Design review of the part built by this model. Coordinates are the model's own, in mm. Face numbers are marked on the shaded views. A direction names the side the tool comes from. Round coordinates to 2 decimals unless told otherwise and drop trailing zeros. Loops run counter-clockwise (first coordinate to the right, second up) from the corner with the lowest first, then second, coordinate; pieces in that order, holes last. Notation, with made-up numbers: (43, -31.75) -> (93, -31.75) arc R25 ccw to (93, -14.75) -> close; hole circle Ø3 at (-32, -31.75). An arc over 180 degrees is marked (long way). Use a Markdown table: item, result. Add a question column.
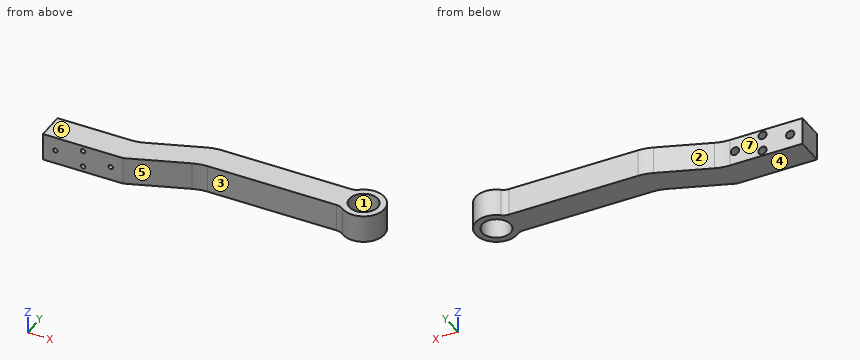
from build123d import *

# Parameters (mm, degrees)
MODEL_R             = 10.3
EXTRUDE_1_DEPTH     = 20
SKETCH_2_R          = 1.6
CUT_EXTRUDE_1_DEPTH = 20
SKETCH_3_R          = 3
CUT_EXTRUDE_2_DEPTH = 8.5


with BuildPart() as part:
    # Model → 凸台-拉伸1 (new body)
    with BuildSketch(Plane.XY):
        with BuildLine():
            Line((125.228900422, 213.510087452), (183.228900422, 213.510087452))
            Line((183.228900422, 213.510087452), (225.242736582, 228.801873242))
            ThreePointArc((225.242736582, 228.801873242), (230.293895552, 230.155327209), (235.503340882, 230.611094618))
            Line((235.503340882, 230.611094618), (328.909813266, 230.611094618))
            ThreePointArc((328.909813266, 230.611094618), (331.547600788, 230.163715156), (333.89036532, 228.871613865))
            ThreePointArc((333.89036532, 228.871613865), (358.22890041, 240.609493061), (333.891295649, 252.349301102))
            ThreePointArc((333.891295649, 252.349301102), (331.548694356, 251.057478239), (328.911168476, 250.610215048))
            Line((328.911168476, 250.610215048), (235.503478715, 250.611047476))
            ThreePointArc((235.503478715, 250.611047476), (230.293897677, 250.15530328), (225.242607062, 248.8018261))
            Line((225.242607062, 248.8018261), (188.1996953, 235.319308829))
            ThreePointArc((188.1996953, 235.319308829), (183.14853633, 233.965854862), (177.939091, 233.510087452))
            Line((177.939091, 233.510087452), (125.228900422, 233.510087452))
            Line((125.228900422, 233.510087452), (125.228900422, 213.510087452))
        make_face()
        with Locations((343.228900422, 240.610087452)):
            Circle(MODEL_R, mode=Mode.SUBTRACT)
    extrude(amount=EXTRUDE_1_DEPTH)

    # 草图2 → 切除-拉伸1 (cut)
    with BuildSketch(Plane.XZ.offset(-213.510087452)):
        with Locations((134.228900422, 10)):
            Circle(SKETCH_2_R)
        with Locations((174.228900422, 10)):
            Circle(SKETCH_2_R)
        with Locations((154.228900422, 16)):
            Circle(SKETCH_2_R)
        with Locations((154.228900422, 4)):
            Circle(SKETCH_2_R)
    extrude(amount=-CUT_EXTRUDE_1_DEPTH, mode=Mode.SUBTRACT)

    # 草图3 → 切除-拉伸2 (cut)
    with BuildSketch(Plane(origin=(0, 233.510087452, 0), x_dir=(1, 0, 0), z_dir=(0, 1, 0))):
        with Locations(Location((134.228900422, -10, 0), (0, 0, 270))):
            Circle(SKETCH_3_R)
        with Locations(Location((154.228900422, -4, 0), (0, 0, 270))):
            Circle(SKETCH_3_R)
        with Locations(Location((154.228900422, -16, 0), (0, 0, 270))):
            Circle(SKETCH_3_R)
        with Locations(Location((174.228900422, -10, 0), (0, 0, 270))):
            Circle(SKETCH_3_R)
    extrude(amount=-CUT_EXTRUDE_2_DEPTH, mode=Mode.SUBTRACT)


solid = part.part
1. Consider section B-B on x = 260. State the section outline as (y, z) points, plus the area to 3 significant figures.
2. Mouldability with a two-part tool opening along X and no side actions: class the marked faces 1, 2, 3 and 4 as +X half, -X half, draft (parallel to the pull), parting line (faces both ways), or undercut.
3. Insertion check: P1, Ø6, axis at x = 263, z = 11.5, coming from the -Y side; P2, Ø5, axis at x = 174.23, z = 10, coming from the +Y side; P3, Ø8, axis at y = 229.5, z = 16.5, coming from the +X side. Each pin has a flat end and moves straight along its axis. Give the tip position at first contact, or say it passes through.
4. Consider section A-A on y = 245. State the section outline as (x, z) points, plus the area to 3 significant figures.
5. Consider section C-C on x = 218. State the section outline as (y, z) points.
6. For the marked faces 5, 6 and 7, list the 3-axis set-ups (+Z, -Z, +X, -X, +Y, -Y) from which the entire face can be reached by the end or side of a thin tool; tool diameter is ignored.
7. To check wall thickness, follow probe 1 along X at (y, z) = (231.5, 6.5); probe 2 along Y at (x, z) = (292, 3.25); probe 3 along Y at (x, z) = (148, 11). State the ranges of each line that lie inside material, in increasing order. Write a range as from..to.
Verdict:
| question | item | result |
|---|---|---|
| 1 | outline | (230.61, 0) -> (250.61, 0) -> (250.61, 20) -> (230.61, 20) -> close |
| 1 | area | 400 mm² |
| 2 | face 1 | undercut |
| 2 | face 2 | -X half |
| 2 | face 3 | undercut |
| 2 | face 4 | draft |
| 3 | P1 | stops at y = 230.61 |
| 3 | P2 | stops at y = 225.01 |
| 3 | P3 | stops at x = 356.44 |
| 4 | outline | (214.8, 0) -> (333.91, 0) -> (333.91, 20) -> (214.8, 20) -> close; (352.55, 0) -> (357.57, 0) -> (357.57, 20) -> (352.55, 20) -> close |
| 4 | area | 2,480 mm² |
| 5 | outline | (226.17, 0) -> (246.17, 0) -> (246.17, 20) -> (226.17, 20) -> close |
| 6 | face 5 | +Z, -Z, -Y |
| 6 | face 6 | +Z, +X, -X, +Y, -Y |
| 6 | face 7 | +Z, -Z, -X, +Y |
| 7 | probe 1 | x = 125.23..152.57, 155.89..338.42, 348.03..355.15 |
| 7 | probe 2 | y = 230.61..250.61 |
| 7 | probe 3 | y = 213.51..233.51 |
